Here's how the part is built. I have some questions about the finished solid (model axes, mm). Round coordinates to 2 decimals unless told otherwise and drop trailing zeros. Write each loop counter-clockwise with the first axis right and the second up, starting at its lowest first coordinate (ties: lowest second). Pieces come first, ordered by that corner, then holes. Notation, with made-up numbers: (9, 79) - (29, 79) arc R23 cw to (29, 115) - close; hole circle Ø6 at (-35, 75.25). An arc over 180 degrees is marked (long way). Use one line per item in the form item = value. Start each with the question number.
1. I want a section at A-A, the plane z = 2.75. List the corners of the cut face in (x, y) for me, plus the area to 3 significant figures.
2. If I drill on line 1 along X through (y, z) = (-8, 2.25); line 2 along X through (y, z) = (-6.5, -7.5); line 3 along Y through (x, z) = (-299, 2.5), over which ranges is the centre line in solid material (lowest first)?
3. Will this pin go through, and if not, where does the flat tip stop? pin 1 (12 mm diameter, centred on x = 307.25, y = 0, fed in from -Z) (1 decimal).
4. We'd pull the mould along X, two halves only. Please class faces 1 (the flat face through (-327.569, 0, 1)), 2 (the flat face through (-5, 25.4, 1)), 3 (the cylindrical face through (315.3, -6.2, 1.1)): +X half, -X half, draft (parallel to the pull), parting line (faces both ways), or undercut.
5. I want a section at B-B, the plane y = 0. List the corners of the cut face in (x, z) for me, plus the area to 3 significant figures.
```python
from build123d import *

# Parameters (mm, degrees)
SKETCH1_W           = 81.89214
SKETCH1_H           = 6.35
BOSS_EXTRUDE1_DEPTH = 2.54
SKETCH3_R           = 1.27
CUT_EXTRUDE1_DEPTH  = 42.147452818
SCALE1_SCALE        = 8


with BuildPart() as part:
    # Sketch1 → Boss-Extrude1 (new body)
    with BuildSketch(Plane.XY):
        Rectangle(SKETCH1_W, SKETCH1_H)
    extrude(amount=BOSS_EXTRUDE1_DEPTH)

    # Sketch3 → Cut-Extrude1 (cut, through all)
    with BuildSketch(Plane.XY):
        with Locations((-38.40607, 0)):
            Circle(SKETCH3_R)
    cut_extrude1 = extrude(amount=CUT_EXTRUDE1_DEPTH, mode=Mode.SUBTRACT)

    # Mirror1: Cut-Extrude1 across plane
    add(cut_extrude1.mirror(Plane(origin=(0, 0, 0), x_dir=(0, 0, 1), z_dir=(1, 0, 0))), mode=Mode.SUBTRACT)


with BuildPart() as part_1:
    # Scale1: scaled about (0, 0, 1.27)
    add(part.part.scale(SCALE1_SCALE).moved(Location((0, 0, -8.89))))


solid = part_1.part
```
Model answer:
q1.outline = (-327.57, -25.4) - (327.57, -25.4) - (327.57, 25.4) - (-327.57, 25.4) - close; hole circle Ø20.32 at (-307.25, 0); hole circle Ø20.32 at (307.25, 0)
q1.area = 32,600 mm2
q2.line_1 = -327.57 to -313.51, -300.99 to 300.99, 313.51 to 327.57
q2.line_2 = -327.57 to -315.06, -299.44 to 299.44, 315.06 to 327.57
q2.line_3 = -25.4 to -5.93, 5.93 to 25.4
q3.pin_1 = through
q4.face_1 = -X half
q4.face_2 = draft
q4.face_3 = undercut
q5.outline = (-327.57, -8.89) - (-317.41, -8.89) - (-317.41, 11.43) - (-327.57, 11.43) - close; (-297.09, -8.89) - (297.09, -8.89) - (297.09, 11.43) - (-297.09, 11.43) - close; (317.41, -8.89) - (327.57, -8.89) - (327.57, 11.43) - (317.41, 11.43) - close
q5.area = 12,500 mm2
